Autodesk Inventor part; units mm, degrees
ref_plane "YZ Plane" through (0, 0, 0) normal (1, 0, 0) x (0, 1, 0)
ref_plane "XZ Plane" through (0, 0, 0) normal (0, 1, 0) x (-1, 0, 0)
ref_plane "XY Plane" through (0, 0, 0) normal (0, 0, 1) x (1, 0, 0)
sketch "Sketch1" plane through (0, 0, 0) normal (0, 1, 0) x (-1, 0, 0)
  line L0 (0, 0) -> (304.8, 0)
  line L1 (304.8, 0) -> (304.8, -609.6)
  line L2 (304.8, -609.6) -> (0, -609.6)
  line L3 (0, -609.6) -> (0, 0)
  dimension "d0" = 609.6
  dimension "d1" = 304.8
extrude "Plate1" add sketch "Sketch1" along normal blind 3.175
sketch "Sketch2" plane through (-3.175, 0, -609.6) normal (1, 0, 0) x (0, 1, 0)
  line L0 (0, 609.6) -> (0, 0)
  line L1 (0, 0) -> (101.6, 0)
  line L2 (101.6, 0) -> (101.6, 609.6)
  line L3 (101.6, 609.6) -> (0, 609.6)
edge flange "Flange1" height 101.6 angle 90 thickness 3.175 bend radius 3.175 thickness toward (1, 0, 0) relief tear relief width 3.175 relief depth 1.5875 edges at (0, 3.175, -304.8) wall of the first edge with corners at (-3.175, 0, 0) (-3.175, 0, -609.6) (-3.175, 101.6, -609.6) (-3.175, 101.6, 0)
bend "Bend1"
corner "Corner1"
chamfer "Chamfer1" distance 12.7 angle 45 2 edges at (-304.8, 1.5875, -609.6) (-304.8, 1.5875, 0)
ref_plane "Work Plane1" through (-6.35, 0, -508) normal (0, 0, -1) x (-1, 0, 0)
sketch "Sketch3" plane through (-6.35, 0, -508) normal (0, 0, -1) x (-1, 0, 0)
  line L0 (-3.175, 6.35) -> (-3.175, 101.6)
  line L1 (-3.175, 15.875) -> (9.525, 3.175)
  line L2 (285.75, 3.175) -> (0, 3.175)
  line L3 (161.925, 3.175) -> (-3.175, 92.075)
  line L4 (-3.175, 92.075) -> (-3.175, 15.875)
  line L5 (9.525, 3.175) -> (161.925, 3.175)
  point P0 (-6.35, 0)
  dimension "d17" = 152.4
  dimension "d18" = 76.2
  dimension "d19" = 12.7
  dimension "d20" = 135
sheet face with bend "Face2" sketch "Sketch3" thickness 3.175 toward (0, 0, -1) bend radius 3.175
bend "Bend2"
ref_plane "Work Plane2" through (-6.35, 0, -304.8) normal (0, 0, -1) x (-1, 0, 0)
mirror "Mirror1" about plane through (-6.35, 0, -304.8) normal (0, 0, -1)
equation "\"d2\" = Thickness"
equation "\"d3\" = BendReliefWidth"
equation "\"d4\" = BendReliefDepth"
equation "\"d5\" = MinimumRemnant"
equation "\"d6\" = TransitionRadius"
equation "\"d9\" = BendRadius"
equation "\"d10\" = CornerReliefSize"
equation "\"d11\" = GapSize"
equation "\"d12\" = JacobiRadiusSize"
equation "\"d21\" = BendRadius"
equation "\"d22\" = BendReliefWidth"
equation "\"d24\" = MinimumRemnant"
equation "\"d23\" = BendReliefDepth"
equation "\"d25\" = TransitionRadius"
equation "\"BendRadius\" = Thickness"
equation "\"BendReliefWidth\" = Thickness"
equation "\"BendReliefDepth\" = 0.5 * Thickness"
equation "\"CornerReliefSize\" = 4 * Thickness"
equation "\"MinimumRemnant\" = 2 * Thickness"
equation "\"TransitionRadius\" = BendRadius"
equation "\"JacobiRadiusSize\" = BendRadius"
equation "\"GapSize\" = Thickness"
properties part number "21015-22-1-6- Work Shelves" material "Steel, Carbon"
Can you work these out from the model? Positions are in its coordinate system, mm. A direction names the side the tool comes from. Round coordinates to 2 decimals unless told otherwise and drop trailing zeros. Loops run counter-clockwise (first coordinate to the right, second up) from the corner with the lowest first, then second, coordinate; pieces in that order, holes last.
Item 1: Suppose I cut it at A-A, the plane y = 52. Write out the boundary of the cut face in (x, z) (3 decimals), then the cut area to 3 significant figures.
Item 2: Suppose I cut it at B-B, the plane z = -442.5. Write out the boundary of the cut face in (x, y) (3 decimals), then the cut area to 3 significant figures.
Item 3: Will these pins go through, and if not, where does the flat tip stop? pin 1 Ø10 at (y, z) = (26, -212) entering from -X (3 decimals); pin 2 Ø3 at (x, z) = (-111, -544.5) entering from +Y (3 decimals); pin 3 Ø6 at (x, y) = (-112, 36.5) entering from -Z (3 decimals).
Item 4: Suppose I cut it at C-C, the plane x = -73. Write out the boundary of the cut face in (y, z) (3 decimals), then the cut area to 3 significant figures.
Item 5: Which directions (+Z, -Z, +X, -X, +Y, -Y) give clear straight access to the entire face, cutting with the end or side of a thin tool? Please do faces 1 (the flat face through (-48, 28, -511.175)), 2 (the flat face through (-50, 28, -98.425)), 3 (the flat face through (-48, 28, -508)).
Item 6: If we mould it in two halves opening along Z, with no side actions, what happens to faces 4 (the flat face through (-145, 2, 0)), 5 (the flat face through (-50, 28, -101.6)), 6 (the flat face through (-84.569, 48.247, -100.035)), 7 (the flat face through (-3.175, 53, -309))? For each: +Z half, -Z half, draft (parallel to the pull), parting line (faces both ways), or undercut.
Item 7: Suppose I cut it at D-D, the plane x = -244.5. Write out the boundary of the cut face in (y, z) (3 decimals).
Item 8: Please list where these lines run through material, in increasing order: L1, parallel to Y at x = -198.5, z = -309.5 (3 decimals); L2, parallel to X at y = 22.5, z = -80.5 (3 decimals); L3, parallel to X at y = 16.5, z = -100.
Reported:
1. outline: (-77.6, -511.175) - (-3.175, -511.175) - (-3.175, -609.6) - (0, -609.6) - (0, 0) - (-3.175, 0) - (-3.175, -98.425) - (-77.6, -98.425) - (-77.6, -101.6) - (-3.175, -101.6) - (-3.175, -508) - (-77.6, -508) - close
1. area: 2,410 mm2
2. outline: (-304.8, 0) - (-6.35, 0) arc R6.35 ccw to (0, 6.35) - (0, 101.6) - (-3.175, 101.6) - (-3.175, 6.35) arc R3.175 cw to (-6.35, 3.175) - (-304.8, 3.175) - close
2. area: 1,270 mm2
3. pin 1: stops at x = -3.175
3. pin 2: stops at y = 3.175
3. pin 3: stops at z = -511.175
4. outline: (0, -609.6) - (3.175, -609.6) - (3.175, -511.175) - (54.477, -511.175) - (54.477, -508) - (3.175, -508) - (3.175, -101.6) - (54.477, -101.6) - (54.477, -98.425) - (3.175, -98.425) - (3.175, 0) - (0, 0) - close
4. area: 2,260 mm2
5. face 1: -Z, -X, +Y
5. face 2: +Z, -X, +Y
5. face 3: -X, +Y
6. face 4: +Z half
6. face 5: undercut
6. face 6: draft
6. face 7: undercut
7. outline: (0, -609.6) - (3.175, -609.6) - (3.175, 0) - (0, 0) - close
8. L1: y = 0 to 3.175
8. L2: x = -3.175 to 0
8. L3: x = -143.53 to 0
